```python
from build123d import *

# Parameters (mm, degrees)
F0_W     = 30.2
F0_H     = 82.2
F1_DEPTH = 5
F2_W     = 20.2
F2_H     = 72.2
F3_DEPTH = 5
F4_SIZE  = 2
F5_W     = 2
F5_H     = 4.2
F6_DEPTH = 5
F7_W     = 4.2
F7_H     = 1
F8_DEPTH = 28.2
F9_R     = 2


with BuildPart() as f1:
    # F0 (on Top) → F1 (new body)
    with BuildSketch(Plane.XY):
        with Locations((15.1, -41.1)):
            Rectangle(F0_W, F0_H)
    extrude(amount=F1_DEPTH)

    # F2 (on face) → F3 (join)
    with BuildSketch(Plane.XY.offset(5)):
        with Locations((15.1, -41.1)):
            Rectangle(F2_W, F2_H)
    extrude(amount=F3_DEPTH)

    # F4
    f4_edges = [f1.edges().sort_by_distance(p)[0] for p in [
        (15.1, -5, 10),
        (5, -41.1, 10),
        (15.1, -77.2, 10),
        (25.2, -41.1, 10),
    ]]
    chamfer(f4_edges, length=F4_SIZE)

    # F5 (on face) → F6 (cut, through all)
    with BuildSketch(Plane.XY.offset(5)):
        with Locations((1, -41.1)):
            Rectangle(F5_W, F5_H)
        with Locations((29.2, -41.1)):
            Rectangle(F5_W, F5_H)
    extrude(amount=-F6_DEPTH, mode=Mode.SUBTRACT)

    # F7 (on Right) → F8 (cut, through all)
    with BuildSketch(Plane.YZ):
        with Locations((-41.1, 0.5)):
            Rectangle(F7_W, F7_H)
    extrude(amount=F8_DEPTH, mode=Mode.SUBTRACT)

    # F9
    f9_edges = [f1.edges().sort_by_distance(p)[0] for p in [
        (2, -41.1, 1),
        (28.2, -41.1, 1),
    ]]
    fillet(f9_edges, radius=F9_R)


solid = f1.part
```
Verification items for the finished model (mm, model axes). A direction names the side the tool comes from. Round coordinates to 2 decimals unless told otherwise and drop trailing zeros. Write each loop counter-clockwise with the first axis right and the second up, starting at its lowest first coordinate (ties: lowest second). Pieces come first, ordered by that corner, then holes.
1. Scan lines: L1, parallel to Z at x = 1, y = -50; L2, parallel to X at y = -10, z = 6; L3, parallel to Y at x = 5.5, z = 7.5. Record each from-to range of solid material in increasing order.
2. Draft check along Y on faces 1 (the flat face through (0, -63, 2)), 2 (the flat face through (15, -82.2, 2)), 3 (the flat face through (28.2, -41, 4)), 4 (the flat face through (2, -41, 4)). Enter one of: +Y half, -Y half, draft (parallel to the pull), parting line (faces both ways), or undercut.
3. Section check D-D on x = 3. Enter the section's corners in (y, z), plus the area to 3 significant figures.
4. Access from +Z, -Z, +X, -X, +Y, -Y to the whole of each face (thin tool, end or side, straight path). Record for faces 5 (the flat face through (15, -41, 1)), 6 (the flat face through (15, -5, 6)), 7 (the cylindrical face through (2.6, -41.13, 1.57)), 8 (the flat face through (14.9, -39, 0.3)), 9 (the flat face through (5, -42, 6)).
5. Section check C-C on z = 6.75. Enter the section's corners in (x, y), plus the area to 3 significant figures.
6. Section check B-B on y = -17.5. Enter the section's corners in (x, z).
7. Section check A-A on x = 20. Enter the section's corners in (y, z).
8. Gauge pin test, flat ends, axial feed: P1, Ø1.5, axis at y = -26.5, z = 6.5, coming from the +X side; P2, Ø2, axis at x = 20.5, z = 7, coming from the -Y side; P3, Ø1, axis at y = -40.5, z = 4, coming from the +X side. Record the tip position at first contact, or that the pin passes through.
Answer:
1. L1: z = 0 to 5
1. L2: x = 5 to 25.2
1. L3: y = -77.2 to -5
2. face 1: draft
2. face 2: -Y half
2. face 3: undercut
2. face 4: undercut
3. outline: (-82.2, 0) - (-43.2, 0) - (-43.2, 1.27) - (-39, 1.27) - (-39, 0) - (0, 0) - (0, 5) - (-82.2, 5) - close
3. area: 406 mm2
4. face 5: -Z, +X, -X
4. face 6: +Z, +X, -X, +Y
4. face 7: -Z, -X
4. face 8: -Z
4. face 9: +Z, -X, +Y, -Y
5. outline: (5, -77.2) - (25.2, -77.2) - (25.2, -5) - (5, -5) - close
5. area: 1,460 mm2
6. outline: (0, 0) - (30.2, 0) - (30.2, 5) - (25.2, 5) - (25.2, 8) - (23.2, 10) - (7, 10) - (5, 8) - (5, 5) - (0, 5) - close
7. outline: (-82.2, 0) - (-43.2, 0) - (-43.2, 1) - (-39, 1) - (-39, 0) - (0, 0) - (0, 5) - (-5, 5) - (-5, 8) - (-7, 10) - (-75.2, 10) - (-77.2, 8) - (-77.2, 5) - (-82.2, 5) - close
8. P1: stops at x = 25.2
8. P2: stops at y = -77.2
8. P3: stops at x = 28.2
